Work out the finished part from the listing and answer in its coordinate system (mm). A direction names the side the tool comes from. Coordinates: 2 decimals unless noted, no trailing zeros. Write each loop counter-clockwise with the first axis right and the second up, starting at its lowest first coordinate (ties: lowest second). Pieces come first, ordered by that corner, then holes. Notation, with made-up numbers: (48.25, 81.5) - (55.25, 81.5) arc R23 cw to (55.25, 107.5) - close; hole circle Ø6 at (15.25, 46). An arc over 180 degrees is marked (long way). Use one line per item in the form item = value. Start each with the question number.
Item 1: Determine the mould class of faces 4 (the flat face through (-32, 0, -1)), 5 (the cylindrical face through (45.99, 9.16, -46.05)), 6 (the cylindrical face through (-38.43, 9.16, -40.79)) for opening direction X: released by +X, released by -X, zero draft, split by the parting line, or undercut.
Item 2: Given pin 1 (3 mm diameter, centred on x = 7, y = 3, fed in from +Z); pin 2 (2.5 mm diameter, centred on x = 40.513, z = -40.513, fed in from -Y); pin 3 (2 mm diameter, centred on y = 3.5, z = 10.5, fed in from +X), each flat-ended and moving along its own axis, determine where each tip first touches the part or whether it passes through.
Item 3: A cutting plane is placed at B-B (z = 0). Write down the section's boundary in (x, y), then the cut area to 3 significant figures.
Item 4: Consider probe 1 along Y at (x, z) = (43, -9); probe 2 along X at (y, z) = (4.5, 0); probe 3 along Z at (x, y) = (-5.5, 5.75). Determine where each line is inside the solid, lowest interval first.
Item 5: A cutting plane is placed at A-A (x = 0). Write down the section's boundary in (y, z), then the cut area to 3 significant figures.
Item 6: For faces 1 (the cylindrical face through (45.99, 9.16, 46.05)), 2 (the flat face through (-1, 8.969, 43)), 3 (the cylindrical face through (-46.05, 9.16, 45.99)), determine the directions among +Z, -Z, +X, -X, +Y, -Y from which every point of the face is accessible in a straight line to the end or side of a thin tool.
Item 7: A cutting plane is placed at C-C (y = 6.75). Write down the section's boundary in (x, z).
from build123d import *

# Parameters (mm, degrees)
SKETCH1_W           = 94.5
SKETCH1_H           = 94.5
SKETCH1_R           = 27.25
SKETCH1_R_2         = 2.1
BOSS_EXTRUDE1_DEPTH = 9.35
FILLET1_R           = 4.2


with BuildPart() as part:
    # Sketch1 → Boss-Extrude1 (new body)
    with BuildSketch(Plane(origin=(0, 0, 0), x_dir=(1, 0, 0), z_dir=(0, 1, 0))):
        Rectangle(SKETCH1_W, SKETCH1_H)
        with Locations(Location((0, 0, 0), (0, 0, 270))):
            Circle(SKETCH1_R, mode=Mode.SUBTRACT)
        with Locations(Location((-40.513, 40.513, 0), (0, 0, 270))):
            Circle(SKETCH1_R_2, mode=Mode.SUBTRACT)
        with Locations(Location((40.513, 40.513, 0), (0, 0, 270))):
            Circle(SKETCH1_R_2, mode=Mode.SUBTRACT)
        with Locations(Location((40.513, -40.513, 0), (0, 0, 270))):
            Circle(SKETCH1_R_2, mode=Mode.SUBTRACT)
        with Locations(Location((-40.513, -40.513, 0), (0, 0, 270))):
            Circle(SKETCH1_R_2, mode=Mode.SUBTRACT)
    extrude(amount=BOSS_EXTRUDE1_DEPTH)

    # Sketch3 → Cut-Revolve1 (revolve, cut)
    with BuildSketch(Plane.XY, mode=Mode.PRIVATE) as cut_revolve1_sk:
        Polygon((-47.25, 8.969), (-35, 8.969), (-35, 0.381), (-47.25, 0.381), (-68.714160929, 0.381), (-68.714160929, 8.969), align=None)
    revolve(cut_revolve1_sk.sketch.rotate(Axis((0, 9.35, 0), (0, -1, 0)), 270), axis=Axis((0, 9.35, 0), (0, -1, 0)), mode=Mode.SUBTRACT)

    # Fillet1
    fillet1_edges = [part.edges().sort_by_distance(p)[0] for p in [
        (0, 0, -27.25),
        (0, 9.35, -27.25),
        (0, 0.381, -35),
        (0, 8.969, -35),
        (47.25, 9.1595, 47.25),
        (-47.25, 9.1595, 47.25),
        (-47.25, 9.1595, -47.25),
        (47.25, 9.1595, -47.25),
    ]]
    fillet(fillet1_edges, radius=FILLET1_R)


solid = part.part
Answer:
q1.face_4 = zero draft
q1.face_5 = released by +X
q1.face_6 = undercut
q2.pin_1 = 35.69
q2.pin_2 = through
q2.pin_3 = 34.04
q3.outline = (-47.25, 0) - (-31.45, 0) arc R4.2 ccw to (-27.25, 4.2) - (-27.25, 5.15) arc R4.2 ccw to (-31.45, 9.35) - (-47.25, 9.35) - (-47.25, 8.97) - (-39.2, 8.97) arc R4.2 cw to (-35, 4.77) - (-35, 4.58) arc R4.2 cw to (-39.2, 0.38) - (-47.25, 0.38) - close; (27.25, 4.2) arc R4.2 ccw to (31.45, 0) - (47.25, 0) - (47.25, 0.38) - (39.2, 0.38) arc R4.2 cw to (35, 4.58) - (35, 4.77) arc R4.2 cw to (39.2, 8.97) - (47.25, 8.97) - (47.25, 9.35) - (31.45, 9.35) arc R4.2 ccw to (27.25, 5.15) - close
q3.area = 164 mm²
q4.probe_1 = 0 to 0.38, 8.97 to 9.35
q4.probe_2 = -35 to -27.25, 27.25 to 35
q4.probe_3 = -34.68 to -26.73, 26.73 to 34.68
q5.outline = (0, -47.25) - (0.38, -47.25) - (0.38, -39.2) arc R4.2 cw to (4.58, -35) - (4.77, -35) arc R4.2 cw to (8.97, -39.2) - (8.97, -47.25) - (9.35, -47.25) - (9.35, -31.45) arc R4.2 ccw to (5.15, -27.25) - (4.2, -27.25) arc R4.2 ccw to (0, -31.45) - close; (0, 31.45) arc R4.2 ccw to (4.2, 27.25) - (5.15, 27.25) arc R4.2 ccw to (9.35, 31.45) - (9.35, 47.25) - (8.97, 47.25) - (8.97, 39.2) arc R4.2 cw to (4.77, 35) - (4.58, 35) arc R4.2 cw to (0.38, 39.2) - (0.38, 47.25) - (0, 47.25) - close
q5.area = 164 mm²
q6.face_1 = +Z, +X, +Y
q6.face_2 = none
q6.face_3 = +Z, -X, +Y
q7.outline = circle Ø70.99 at (0, 0); hole circle Ø55.13 at (0, 0)
